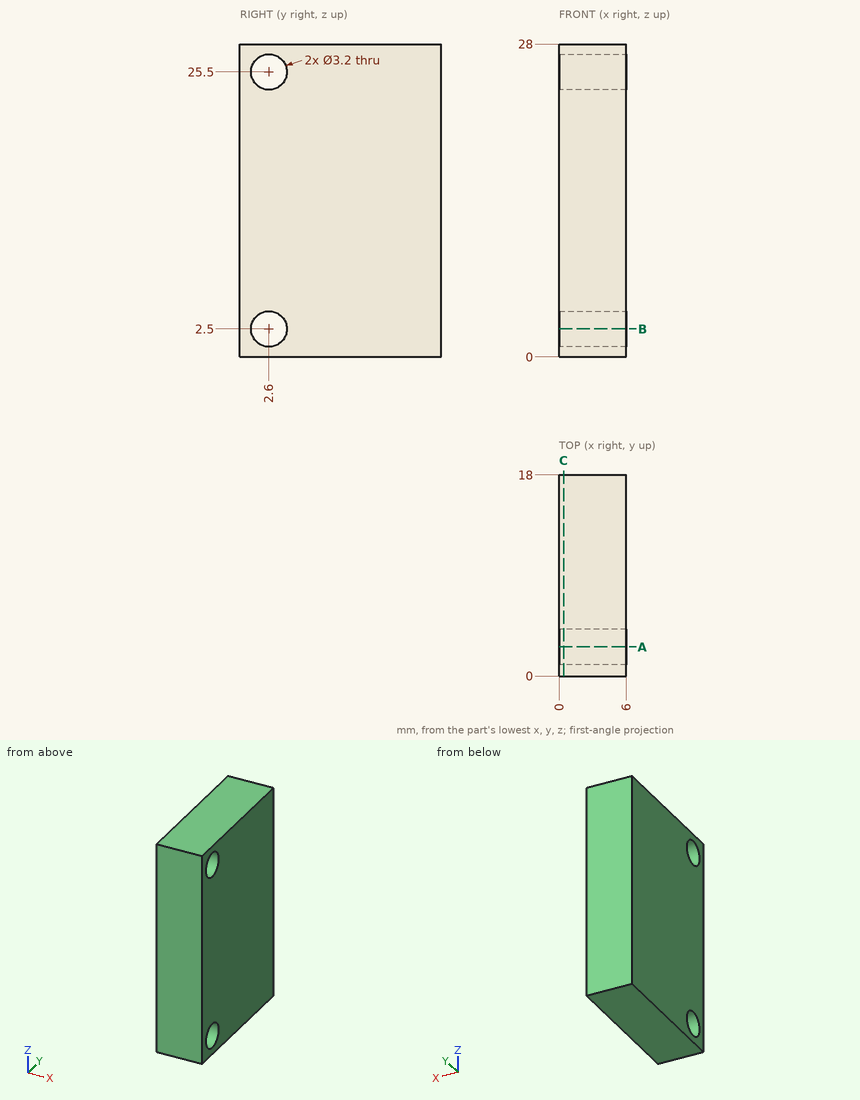
Can you work these out from the drawing? Everything is in mm from the part's minimum corner. Coordinates: 2 decimals unless noted, no trailing zeros. Write each loop counter-clockwise with the first axis right and the second up, starting at its lowest first coordinate (ties: lowest second). Pieces come first, ordered by that corner, then holes. Notation, with made-up numbers: (43.25, -26) -> (95.25, -26) arc R19 cw to (95.25, -12) -> close; hole circle Ø8 at (-32, -38). An arc over 180 degrees is marked (long way). Write each question's results on one line, items separated by ' | '. Start each with the question number.
Q1. Imagine slicing it at C-C (x = 0.4). Write out the boundary of the cut face in (y, z), then the cut area to 3 significant figures.
Q2. Imagine slicing it at B-B (z = 2.5). Write out the boundary of the cut face in (x, y).
Q3. Imagine slicing it at A-A (y = 2.6). Write out the boundary of the cut face in (x, z).
Q4. If I drill on probe 1 along Z at (x, y) = (4.6, 2.5); probe 2 along Y at (x, z) = (4.4, 2.5); probe 3 along Z at (x, y) = (4.65, 1.25), over which ranges is the centre line in solid material (lowest first)?
Taken from the geometry:
1) outline: (0, 0) -> (18, 0) -> (18, 28) -> (0, 28) -> close; hole circle Ø3.2 at (2.6, 2.5); hole circle Ø3.2 at (2.6, 25.5) | area: 488 mm^2
2) outline: (0, 0) -> (6, 0) -> (6, 1) -> (0, 1) -> close; (0, 4.2) -> (6, 4.2) -> (6, 18) -> (0, 18) -> close
3) outline: (0, 0) -> (6, 0) -> (6, 0.9) -> (0, 0.9) -> close; (0, 4.1) -> (6, 4.1) -> (6, 23.9) -> (0, 23.9) -> close; (0, 27.1) -> (6, 27.1) -> (6, 28) -> (0, 28) -> close
4) probe 1: z = 0 to 0.9, 4.1 to 23.9, 27.1 to 28 | probe 2: y = 0 to 1, 4.2 to 18 | probe 3: z = 0 to 1.64, 3.36 to 24.64, 26.36 to 28
